CAD build for the part. Positions are in the model's coordinates, mm. Give positions to 0.01 mm unless a question says otherwise; leave off trailing zeros. Write each loop counter-clockwise with the first axis right and the second up, starting at its lowest first coordinate (ties: lowest second). Pieces come first, ordered by that corner, then holes. Notation, with made-up numbers: (61.25, 85.25) - (93.25, 85.25) arc R8 ccw to (93.25, 99.25) - close; hole circle Ø6 at (-5.75, 77.5). An arc over 180 degrees is marked (long way). Answer as a JSON object with one key per item and string values.
from build123d import *

# Parameters (mm, degrees)
SKETCH1_W           = 35
SKETCH1_H           = 12
SKETCH1_R           = 0.8001
SKETCH1_R_2         = 1.4732
BOSS_EXTRUDE1_DEPTH = 0.2


with BuildPart() as part:
    # Sketch1 → Boss-Extrude1 (new body)
    with BuildSketch(Plane.XY):
        with Locations((17.5, -6)):
            Rectangle(SKETCH1_W, SKETCH1_H)
        with Locations((3.5, -8.3)):
            Circle(SKETCH1_R, mode=Mode.SUBTRACT)
        with Locations((5, -4.5)):
            Circle(SKETCH1_R_2, mode=Mode.SUBTRACT)
        with Locations((30, -4.5)):
            Circle(SKETCH1_R_2, mode=Mode.SUBTRACT)
        with Locations((31.5, -8.3)):
            Circle(SKETCH1_R, mode=Mode.SUBTRACT)
        with BuildLine():
            Line((14.2, -1.795803989), (14.2, -3.575))
            ThreePointArc((14.2, -3.575), (14.214644661, -3.610355339), (14.25, -3.625))
            Line((14.25, -3.625), (20.75, -3.625))
            ThreePointArc((20.75, -3.625), (20.785355339, -3.610355339), (20.8, -3.575))
            Line((20.8, -3.575), (20.8, -1.795803989))
            ThreePointArc((20.8, -1.795803989), (20.520871215, -1.306350833), (21.05, -1.5))
            Line((21.05, -1.5), (21.05, -3.575))
            ThreePointArc((21.05, -3.575), (20.962132034, -3.787132034), (20.75, -3.875))
            Line((20.75, -3.875), (14.25, -3.875))
            ThreePointArc((14.25, -3.875), (14.037867966, -3.787132034), (13.95, -3.575))
            Line((13.95, -3.575), (13.95, -1.5))
            ThreePointArc((13.95, -1.5), (14.479128785, -1.306350833), (14.2, -1.795803989))
        make_face(mode=Mode.SUBTRACT)
        with BuildLine():
            Line((20.477282197, -4.375), (14.522717803, -4.375))
            ThreePointArc((14.522717803, -4.375), (13.95, -4.5), (14.522717803, -4.625))
            Line((14.522717803, -4.625), (20.477282197, -4.625))
            ThreePointArc((20.477282197, -4.625), (21.05, -4.5), (20.477282197, -4.375))
        make_face(mode=Mode.SUBTRACT)
    extrude(amount=BOSS_EXTRUDE1_DEPTH)


solid = part.part
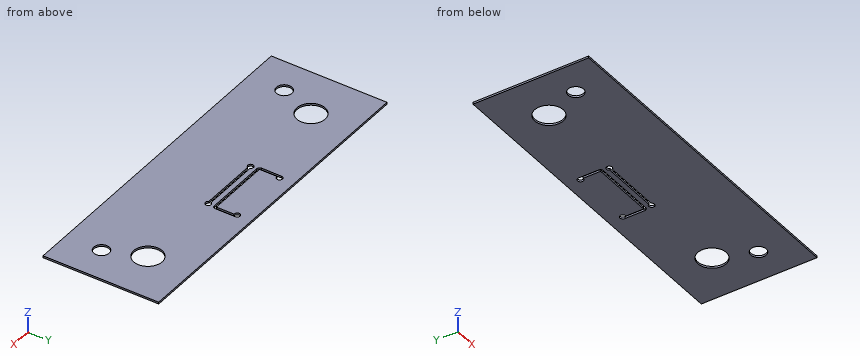
(1) Saw through at A-A, the plane x = 5. Give the cut face in (y, z), and give its area (3 significant figures).
Answer key:
{"outline": "(-12, 0) - (-5.97, 0) - (-5.97, 0.2) - (-12, 0.2) - close; (-3.03, 0) - (0, 0) - (0, 0.2) - (-3.03, 0.2) - close", "area": "1.81 mm²"}
(2) Saw through at C-C, the plane y = -5.5. Give the cut face in (x, z), and give its area (3 significant figures).
Answer key:
{"outline": "(0, 0) - (3.92, 0) - (3.92, 0.2) - (0, 0.2) - close; (6.08, 0) - (28.92, 0) - (28.92, 0.2) - (6.08, 0.2) - close; (31.08, 0) - (35, 0) - (35, 0.2) - (31.08, 0.2) - close", "area": "6.13 mm²"}
(3) Saw through at B-B, the plane z = 0.15. Give the cut face in (x, y) (3 decimals), and give its area (3 significant figures).
Answer key:
{"outline": "(0, -12) - (35, -12) - (35, 0) - (0, 0) - close; hole circle Ø1.6 at (3.5, -8.3); hole circle Ø2.946 at (5, -4.5); hole (13.95, -3.575) arc R0.3 ccw to (14.25, -3.875) - (20.75, -3.875) arc R0.3 ccw to (21.05, -3.575) - (21.05, -1.5) arc R0.3 ccw (long way) to (20.8, -1.796) - (20.8, -3.575) arc R0.05 cw to (20.75, -3.625) - (14.25, -3.625) arc R0.05 cw to (14.2, -3.575) - (14.2, -1.796) arc R0.3 ccw (long way) to (13.95, -1.5) - close; hole (14.523, -4.625) - (20.477, -4.625) arc R0.3 ccw (long way) to (20.477, -4.375) - (14.523, -4.375) arc R0.3 ccw (long way) to start; hole circle Ø2.946 at (30, -4.5); hole circle Ø1.6 at (31.5, -8.3)", "area": "397 mm²"}
(4) Probe L1, parallel to Y at x = 16, z = 0.15 (3 decimals); L2, parallel to X at y = -1.5, z = 0.1; L3, parallel to Y at x = 20.75, z = 0.1 (3 decimals). List the from-to ranges inside material, lowest first. Write a range as [from, to].
Answer key:
{"L1": "y = [-12, -4.625], [-4.375, -3.875], [-3.625, 0]", "L2": "x = [0, 13.95], [14.55, 20.45], [21.05, 35]", "L3": "y = [-12, -4.8], [-4.2, -3.875], [-3.625, -1.8], [-1.2, 0]"}
